```python
from build123d import *

# Parameters (mm, degrees)
SKETCH1_R           = 7
BOSS_EXTRUDE1_DEPTH = 44
SKETCH2_R           = 2.5
CUT_EXTRUDE1_DEPTH  = 10
CUT_EXTRUDE2_START  = -10
SKETCH3_R           = 2.5
CUT_EXTRUDE2_DEPTH  = 10
SKETCH4_R           = 3.5
CUT_EXTRUDE3_DEPTH  = 20
SKETCH5_W           = 18.912740594
SKETCH5_H           = 2.214003862
CUT_EXTRUDE5_DEPTH  = 35


with BuildPart() as part:
    # Sketch1 → Boss-Extrude1 (new body)
    with BuildSketch(Plane.XY):
        Circle(SKETCH1_R)
    extrude(amount=BOSS_EXTRUDE1_DEPTH)

    # Sketch2 → Cut-Extrude1 (cut)
    with BuildSketch(Plane.XY.offset(44)):
        Circle(SKETCH2_R)
    extrude(amount=-CUT_EXTRUDE1_DEPTH, mode=Mode.SUBTRACT)

    # Sketch3 → Cut-Extrude2 (cut)
    with BuildSketch(Plane(origin=(0, 0, 0), x_dir=(-1, 0, 0), z_dir=(0, 0, -1)).offset(CUT_EXTRUDE2_START)):
        with Locations(Location((0, 0, 0), (0, 0, 180))):
            Circle(SKETCH3_R)
    extrude(amount=CUT_EXTRUDE2_DEPTH, mode=Mode.SUBTRACT)

    # Sketch4 → Cut-Extrude3 (cut, symmetric)
    with BuildSketch(Plane(origin=(0, 0, 0), x_dir=(1, 0, 0), z_dir=(0, 1, 0))):
        with Locations(Location((0, -22, 0), (0, 0, 270))):
            Circle(SKETCH4_R)
    extrude(amount=CUT_EXTRUDE3_DEPTH, both=True, mode=Mode.SUBTRACT)

    # Sketch5 → Cut-Extrude5 (cut, symmetric)
    with BuildSketch(Plane(origin=(0, 0, 0), x_dir=(0, 0, -1), z_dir=(1, 0, 0))):
        with Locations((-22, 7)):
            Rectangle(SKETCH5_W, SKETCH5_H)
        with Locations((-22, -7)):
            Rectangle(SKETCH5_W, SKETCH5_H)
    extrude(amount=CUT_EXTRUDE5_DEPTH, both=True, mode=Mode.SUBTRACT)


solid = part.part
```
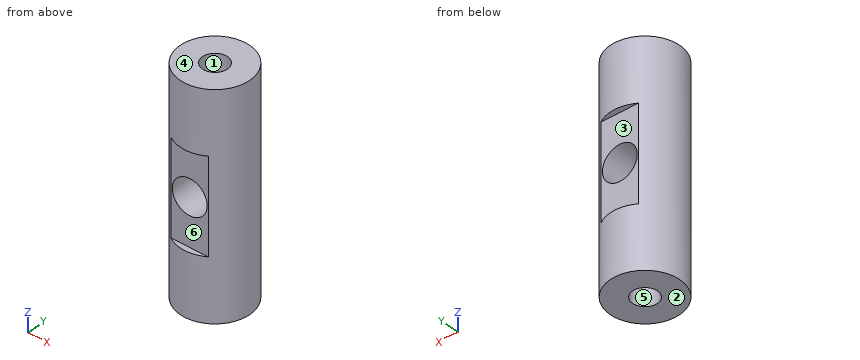
Here's how the part is built. I have some questions about the finished solid (model axes, mm). Face numbers are marked on the shaded views. A direction names the side the tool comes from. Round coordinates to 2 decimals unless told otherwise and drop trailing zeros. Order: outer loops, then holes, each group sorted by start corner. A loop starts at its lowest first (then second) coordinate and runs counter-clockwise, first axis right, second up. Notation, with made-up numbers: M -14.75,5 L 19.25,5 A25 cw 19.25,41 Z; hole C 1.25,13.25 d7. An arc over 180 degrees is marked long. One line per question, with ' | ' between items.
1) I want a section at A-A, the plane x = 0. Write out the boundary of the cut face in (y, z), then the cut area to 3 significant figures.
Working result:
outline: M -7,0 L -2.5,0 L -2.5,10 L 2.5,10 L 2.5,0 L 7,0 L 7,12.54 L 5.89,12.54 L 5.89,18.5 L -5.89,18.5 L -5.89,12.54 L -7,12.54 Z; M -7,31.46 L -5.89,31.46 L -5.89,25.5 L 5.89,25.5 L 5.89,31.46 L 7,31.46 L 7,44 L 2.5,44 L 2.5,34 L -2.5,34 L -2.5,44 L -7,44 Z | area: 392 mm²
2) I need wall thicknesses on line 1 along Y through (x, z) = (0, 4.25); line 2 along Y through (x, z) = (-2.75, 30); line 3 along Z through (x, y) = (2, -4.5). Which ranges of each line are inside material? Lowest first, please.
Working result:
line 1: -7 to -2.5, 2.5 to 7 | line 2: -5.89 to 5.89 | line 3: 0 to 19.13, 24.87 to 44
3) If we mould it in two halves opening along Z, with no side actions, what happens to the marked faces 1, 2 and 3? For each: +Z half, -Z half, draft (parallel to the pull), parting line (faces both ways), or undercut.
Working result:
face 1: draft | face 2: -Z half | face 3: undercut
4) I want a section at C-C, the plane z = 22. Write out the boundary of the cut face in (x, y), then the cut area to 3 significant figures.
Working result:
outline: M -3.78,-5.89 L -3.5,-5.89 L -3.5,5.89 L -3.78,5.89 A7 ccw Z; M 3.5,-5.89 L 3.78,-5.89 A7 ccw 3.78,5.89 L 3.5,5.89 Z | area: 60.1 mm²
5) I want a section at D-D, the plane z = 8. Write out the boundary of the cut face in (x, y), then the cut area to 3 significant figures.
Working result:
outline: C 0,0 d14; hole C 0,0 d5 | area: 134 mm²
6) For the marked faces 4, 5 and 6, which set-ups out of +Z, -Z, +X, -X, +Y, -Y let a thin tool reach every point of the face, with its end or its side?
Working result:
face 4: +Z, +X, -X, +Y, -Y | face 5: -Z | face 6: +X, -X, -Y
7) For pin 1 Ø4 at (x, z) = (4.5, 34) entering from +Y; pin 2 Ø5 at (x, z) = (5.5, 25) entering from +Y; pin 3 Ø3 at (x, y) = (0, 0) entering from +Z, each with a flat end and sliding along its axis, tell me the tip position at first contact or that it passes through.
Working result:
pin 1: y = 6.54 | pin 2: y = 5.89 | pin 3: z = 34
8) I want a section at B-B, the plane y = 0. Write out the boundary of the cut face in (x, z), then the cut area to 3 significant figures.
Working result:
outline: M -7,0 L -2.5,0 L -2.5,10 L 2.5,10 L 2.5,0 L 7,0 L 7,44 L 2.5,44 L 2.5,34 L -2.5,34 L -2.5,44 L -7,44 Z; hole C 0,22 d7 | area: 478 mm²
